Source: CAD feature listing. Evaluate the final solid. Frame: model axes, mm. Face numbers are marked on the shaded views. A direction names the side the tool comes from. Round coordinates to 2 decimals unless told otherwise and drop trailing zeros. Order: outer loops, then holes, each group sorted by start corner. A loop starts at its lowest first (then second) coordinate and runs counter-clockwise, first axis right, second up. Notation, with made-up numbers: (-18.75, 13) - (27.25, 13) arc R16 cw to (27.25, 40) - close; hole circle Ø8 at (32, -8.5). An arc over 180 degrees is marked (long way). Put each result on its own line as item: value. Start each with the question number.
1) Contact query for flat-ended pins moving along their axis: P1, Ø21, axis at x = 51.3, y = 0, coming from the +Z side; P2, Ø2.5, axis at x = 24.1, z = 0, coming from the -Y side; P3, Ø8, axis at x = 41.5, z = 4.5, coming from the +Y side. Output: stop coordinate, or through.
2) Section C-C on z = 11. Output: boundary loops of the cut face in (x, y).
3) Section A-A on x = -24.1. Output: boundary loops of the cut face in (y, z), then the cut area to 3 significant figures.
4) Section B-B on x = 51.3. Output: boundary loops of the cut face in (y, z).
5) Line query: probe 1 along X at (y, z) = (-24.3, 0); probe 2 along Y at (x, z) = (51.3, -23.35); probe 3 along Z at (x, y) = (58, 20). Output: solid intervals per line, ascending. Write a range as [from, to].
6) Section D-D on y = 12. Output: boundary loops of the cut face in (x, z), then the cut area to 3 significant figures.
7) Access query for the marked faces 1 and 2. Directions: +Z, -Z, +X, -X, +Y, -Y. A direction counts if a zero-diameter tool reaches every point of the face in a straight line with its end or side. Return the directions, or none.
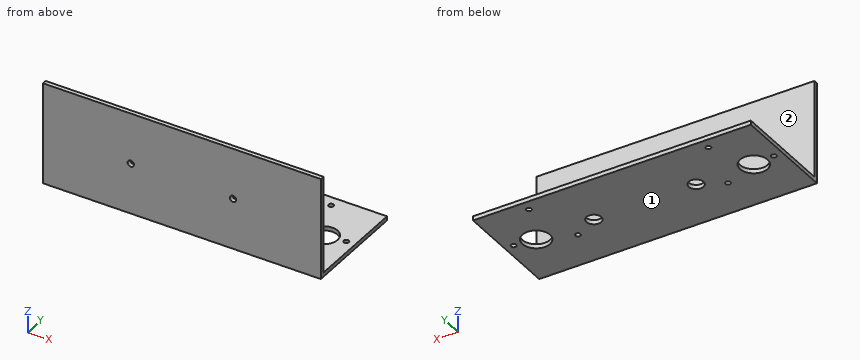
Autodesk Inventor part; units mm, degrees
ref_plane "YZ Plane" through (0, 0, 0) normal (1, 0, 0) x (0, 1, 0)
ref_plane "XZ Plane" through (0, 0, 0) normal (0, 1, 0) x (-1, 0, 0)
ref_plane "XY Plane" through (0, 0, 0) normal (0, 0, 1) x (1, 0, 0)
sketch "Sketch1" plane through (0, 0, 0) normal (1, 0, 0) x (0, 1, 0)
  line L0 (-25, 24) -> (-25, -24)
  line L1 (-25, -24) -> (25, -24)
  line L2 (25, -24) -> (25, -22)
  line L3 (25, -22) -> (-23, -22)
  line L4 (-23, -22) -> (-23, 24)
  line L5 (-23, 24) -> (-25, 24)
extrude "Extrusion1" add sketch "Sketch1" along normal mid plane 131
sketch "Sketch2" plane through (65.5, 25, -24) normal (0, 0, -1) x (-1, 0, 0)
  circle A0 centre (41.4, -25) radius 3.5
  circle A1 centre (89.6, -25) radius 3.5
  dimension "d17" = 7
  dimension "d18" = 7
hole "Hole1" at (24.1, 0, -24) at (-24.1, 0, -24) direction (0, 0, 1) diameter 7 depth 2
sketch "Sketch3" plane through (65.5, 25, -24) normal (0, 0, -1) x (-1, 0, 0)
  line L0 (65.5, -25) -> (14.2, -25)
  line L1 (65.5, -25) -> (116.8, -25)
  circle A0 centre (14.2, -25) radius 9.5
  circle A1 centre (14.2, -25) radius 1.75
  circle A2 centre (116.8, -25) radius 1.75
  dimension "d26" = 51.3
  dimension "d27" = 51.3
  dimension "d28" = 19
  dimension "d29" = 3.5
  dimension "d30" = 3.5
hole "Hole2" at (51.3, 0, -24) at (-51.3, 0, -24) direction (0, 0, 1) diameter 3.5 depth 2
sketch "Sketch5" plane through (-65.5, -23, 24) normal (0, 1, 0) x (1, 0, 0)
  circle A0 centre (41.4, 24) radius 1.2
  circle A1 centre (89.6, 24) radius 1.2
  dimension "d62" = 2.4
  dimension "d63" = 2.4
hole "Hole4" at (-24.1, -23, 0) at (24.1, -23, 0) direction (0, -1, 0) diameter 3 depth 2
sketch "Sketch7" plane through (65.5, 25, -24) normal (0, 0, -1) x (-1, 0, 0)
  circle A0 centre (14.2, -25) radius 1.75
  circle A1 centre (14.2, -25) radius 3.5
  point P0 (65.5, -25)
  dimension "d89" = 7
extrude "Extrusion3" cut sketch "Sketch7" against normal blind 2
sketch "Sketch8" plane through (65.5, 25, -24) normal (0, 0, -1) x (-1, 0, 0)
  circle A0 centre (14.2, -25) radius 3.5
  line L0 (14.2, -25) -> (39.2, -25) construction
  circle A1 centre (19.1497, -20.0503) radius 18.4
  circle A2 centre (19.1497, -20.0503) radius 15.5
  line L1 (14.2, -25) -> (19.1497, -20.0503)
  line L2 (19.1497, -20.0503) -> (36.8274, -2.3726)
  line L3 (36.8274, -2.3726) -> (1.4721, -37.7279)
  line L4 (6.139, -7.0395) -> (32.1605, -33.061)
  circle A3 centre (8.1896, -9.0901) radius 1.2
  circle A4 centre (30.1099, -31.0104) radius 1.2
  circle A5 centre (23.1614, -5.0784) radius 1.2
  circle A6 centre (4.1779, -24.0619) radius 1.2
  circle A7 centre (15.1381, -35.0221) radius 1.2
  circle A8 centre (34.1216, -16.0386) radius 1.2
  point P0 (65.5, -25)
  dimension "d96" = 31
  dimension "d97" = 25
  dimension "d98" = 180
  dimension "d99" = 50
  dimension "d100" = 2.4
  dimension "d101" = 2.4
  dimension "d104" = 2.4
  dimension "d105" = 2.4
  dimension "d106" = 2.4
  dimension "d107" = 2.4
extrude "Extrusion4" cut sketch "Sketch8" against normal blind 2 contours A3 A2 L4 | L4 A2 A3 | A4 A2 L4 | L4 A2 A4 | A6 A2 | A2 A6 | A7 A2 | A2 A7 | A8 A2 | A2 A8 | A5 A2 | A2 A5 | L4 A3 A2 | A2 A3 L4 | L4 A4 A2 | A2 A4 L4
sketch "Sketch9" plane through (65.5, 25, -24) normal (0, 0, -1) x (-1, 0, 0)
  circle A0 centre (34.1216, -16.0386) radius 1.2
  circle A1 centre (8.1896, -9.0901) radius 1.2
  circle A2 centre (15.1381, -35.0221) radius 1.2
  point P0 (65.5, -25)
extrude "Extrusion6" add sketch "Sketch9" against normal blind 2
sketch "Sketch11" plane through (65.5, 25, -24) normal (0, 0, -1) x (-1, 0, 0)
  circle A0 centre (4.1779, -24.0619) radius 1.2
  circle A1 centre (30.1099, -31.0104) radius 1.2
  circle A2 centre (23.1614, -5.0784) radius 1.2
  circle A3 centre (14.2, -25) radius 3.5
  circle A4 centre (116.8, -25) radius 1.75
  line L0 (65.5, -25) -> (65.5, 0)
  line L1 (0, 0) -> (131, 0)
  circle A5 centre (126.8221, -24.0619) radius 1.2
  circle A6 centre (100.8901, -31.0104) radius 1.2
  circle A7 centre (107.8386, -5.0784) radius 1.2
  circle A8 centre (116.8, -25) radius 3.5
extrude "Extrusion7" cut sketch "Sketch11" against normal blind 2 contours A5 | A6 | A7 | A8
sketch "Sketch12" plane through (65.5, 25, -24) normal (0, 0, -1) x (-1, 0, 0)
  circle A0 centre (116.8, -25) radius 3.5
  circle A1 centre (14.2, -25) radius 3.5
  circle A2 centre (14.2, -25) radius 6.5
  circle A3 centre (116.8, -25) radius 6.5
  point P0 (65.5, -25)
  dimension "d116" = 13
  dimension "d117" = 13
extrude "Extrusion8" cut sketch "Sketch12" against normal blind 2
properties part number "drzak_motory"
Answer sheet:
1. P1: z = -22
1. P2: through
1. P3: y = -23
2. outline: (-65.5, -25) - (65.5, -25) - (65.5, -23) - (-65.5, -23) - close
3. outline: (-25, -24) - (-3.5, -24) - (-3.5, -22) - (-23, -22) - (-23, -1.5) - (-25, -1.5) - close; (-25, 1.5) - (-23, 1.5) - (-23, 24) - (-25, 24) - close; (3.5, -24) - (25, -24) - (25, -22) - (3.5, -22) - close
3. area: 172 mm^2
4. outline: (-25, -24) - (-6.5, -24) - (-6.5, -22) - (-23, -22) - (-23, 24) - (-25, 24) - close; (6.5, -24) - (25, -24) - (25, -22) - (6.5, -22) - close
5. probe 1: [-65.5, -25.6], [-22.6, 22.6], [25.6, 65.5]
5. probe 2: [-25, -6.5], [6.5, 25]
5. probe 3: [-24, -22]
6. outline: (-65.5, -24) - (65.5, -24) - (65.5, -22) - (-65.5, -22) - close
6. area: 262 mm^2
7. face 1: -Z, +X, -X, +Y, -Y
7. face 2: +Z, +X, -X, +Y
